Model file for the job. Use its own axes, mm. A direction names the side the tool comes from. Coordinates: 2 decimals unless noted, no trailing zeros. Order: outer loops, then holes, each group sorted by start corner. A loop starts at its lowest first (then second) coordinate and runs counter-clockwise, first axis right, second up.
from build123d import *

# Parameters (mm, degrees)
BOSS_EXTRUDE1_DEPTH = 2
SKETCH3_W           = 10
SKETCH3_H           = 4
CUT_EXTRUDE2_DEPTH  = 67.610809934


with BuildPart() as part:
    # Sketch1 → Boss-Extrude1 (new, symmetric)
    with BuildSketch(Plane(origin=(0, 0, 0), x_dir=(1, 0, 0), z_dir=(0, 1, 0))):
        Polygon((-65, -10), (-50, -10), (-50, -14), (-40, -14), (-40, -10), (-25, -10), (-25, -14), (-7, -14), (-7, -10), (11, -10), (11, -14), (29, -14), (29, -10), (47, -10), (47, -14), (65, -14), (65, -10), (65, 10), (65, 14), (35, 14), (35, 10), (5, 10), (5, 14), (-25, 14), (-25, 10), (-55, 10), (-55, 14), (-65, 14), (-65, 10), align=None)
    extrude(amount=BOSS_EXTRUDE1_DEPTH, both=True)

    # Sketch3 → Cut-Extrude2 (cut, through all)
    with BuildSketch(Plane(origin=(0, 2, 0), x_dir=(1, 0, 0), z_dir=(0, 1, 0))):
        with Locations((-60, 12)):
            Rectangle(SKETCH3_W, SKETCH3_H)
    extrude(amount=-CUT_EXTRUDE2_DEPTH, mode=Mode.SUBTRACT)


solid = part.part
Q1. Drop flat-ended pins along their axis: P1, Ø1.2, axis at x = 2, y = 0.5, coming from the +Z side; P2, Ø2, axis at x = 23.5, y = 0, coming from the -Z side; P3, Ø2, axis at y = 0.5, z = -12, coming from the -X side. Give the stop position or say it passes through.
Established:
P1: stops at z = 10
P2: stops at z = -10
P3: stops at x = -25
Q2. Mould opens along X. For faces 4 (the face through (-7, 0, 12)), 5 (the face through (20, 0, 14)), 6 (the face through (65, 0, 0)), 7 (the face through (-40, 0, 12)) say: pulls with the +X half, pulls with the -X half, needs draft (parallel to the pull), parting line crosses it, or undercut.
Established:
face 4: undercut
face 5: needs draft
face 6: pulls with the +X half
face 7: undercut
Q3. Cut at B-B, the plane y = -0.5. List the corners of the cut face in (x, z).
Established:
outline: (-65, -10) - (-25, -10) - (-25, -14) - (5, -14) - (5, -10) - (35, -10) - (35, -14) - (65, -14) - (65, 14) - (47, 14) - (47, 10) - (29, 10) - (29, 14) - (11, 14) - (11, 10) - (-7, 10) - (-7, 14) - (-25, 14) - (-25, 10) - (-40, 10) - (-40, 14) - (-50, 14) - (-50, 10) - (-65, 10) - close
Q4. Probe line 1 (X direction, y = 1, z = 11.25); line 2 (X direction, y = 0.2, z = -12.5); line 3 (Z direction, x = -40.5, y = -1.45). List the from-to ranges inside material, lowest first.
Established:
line 1: x = -50 to -40, -25 to -7, 11 to 29, 47 to 65
line 2: x = -25 to 5, 35 to 65
line 3: z = -10 to 14
Q5. Cut at A-A, the plane z = -11.25. List the corners of the cut face in (x, y).
Established:
outline: (-25, -2) - (5, -2) - (5, 2) - (-25, 2) - close; (35, -2) - (65, -2) - (65, 2) - (35, 2) - close
Q6. Cut at C-C, the plane x = 25.5. List the corners of the cut face in (y, z).
Established:
outline: (-2, -10) - (2, -10) - (2, 14) - (-2, 14) - close
Q7. Which spindle directions (+Z, -Z, +X, -X, +Y, -Y) get a long thin tool onto all of the face, cutting with end or side? Do faces 1 (the face through (-25, 0, -12)), 2 (the face through (2, 0, 10)), 3 (the face through (20, 0, -10)). Say none if no direction does.
Established:
face 1: -Z, -X, +Y, -Y
face 2: +Z, +Y, -Y
face 3: -Z, +Y, -Y
